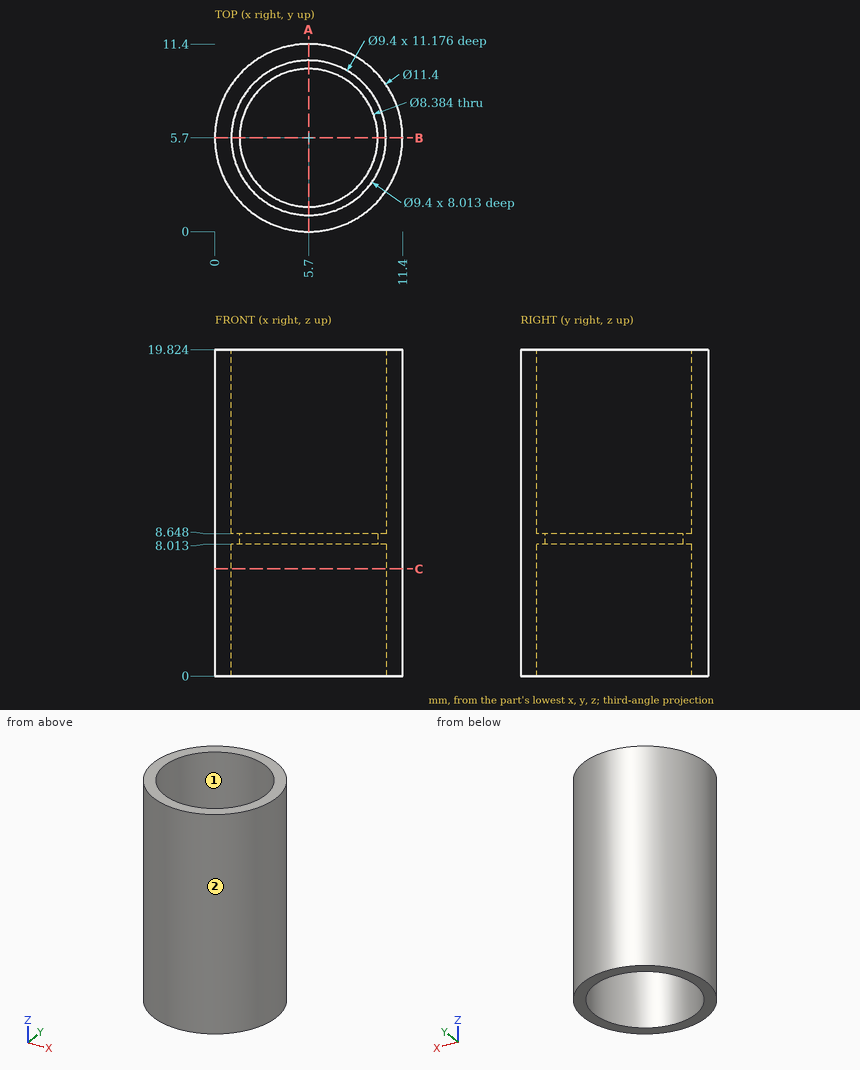
Here's the drawing with two shaded views (mm, measured from the low corner). I have some questions. Coordinates: 2 decimals unless noted, no trailing zeros. Order: outer loops, then holes, each group sorted by start corner. A loop starts at its lowest first (then second) coordinate and runs counter-clockwise, first axis right, second up.
Q1. Suppose I cut it at C-C on z = 6.5. Please give me the cut outline in (x, y).
Q2. Will these pins go through, and if not, where does the flat tip stop? pin 1 (3 mm diameter, centred on x = 9.5, z = 10.5, fed in from +Y); pin 2 (4 mm diameter, centred on y = 1.5, z = 4, fed in from +X); pin 3 (3 mm diameter, centred on y = 2.5, z = 3, fed in from +X).
Q3. Please list where these lines run through material, in increasing order: L1, parallel to X at y = 5.5, z = 13; L2, parallel to Y at x = 5.7, z = 8.25; L3, parallel to Y at x = 8.25, z = 16.
Q4. Suppose I cut it at A-A on x = 5.7. Please give me the cut outline in (y, z), and give its area (3 significant figures).
Q5. Thinking about a two-plate mould opening in Y: for the marked faces 1 and 2, which applies, released by +Y, released by -Y, zero draft, split by the parting line, or undercut?
Answer:
1. outline: circle Ø11.4 at (5.7, 5.7); hole circle Ø9.4 at (5.7, 5.7)
2. pin 1: stops at y = 10.92
2. pin 2: stops at x = 10.96
2. pin 3: stops at x = 11.14
3. L1: x = 0 to 1, 10.4 to 11.4
3. L2: y = 0 to 1.51, 9.89 to 11.4
3. L3: y = 0.6 to 1.75, 9.65 to 10.8
4. outline: (0, 0) - (1, 0) - (1, 8.01) - (1.51, 8.01) - (1.51, 8.65) - (1, 8.65) - (1, 19.82) - (0, 19.82) - close; (9.89, 8.01) - (10.4, 8.01) - (10.4, 0) - (11.4, 0) - (11.4, 19.82) - (10.4, 19.82) - (10.4, 8.65) - (9.89, 8.65) - close
4. area: 40.3 mm2
5. face 1: undercut
5. face 2: split by the parting line
